The listing builds one solid part. Answer for the finished solid, in the listing's coordinates (mm). Coordinates: 2 decimals unless noted, no trailing zeros. Order: outer loops, then holes, each group sorted by start corner. A loop starts at its lowest first (then second) coordinate and runs counter-clockwise, first axis right, second up.
```python
from build123d import *

# Parameters (mm, degrees)
F0_R     = 3.175
F1_DEPTH = 6.35


with BuildPart() as f1:
    # F0 (on Top) → F1 (new body)
    with BuildSketch(Plane.XY):
        Polygon((0, 254), (0, 0), (53.975, 0), (53.975, 25.4), (73.025, 50.8), (73.025, 127), (485.775, 127), (485.775, 50.8), (504.825, 25.4), (504.825, 0), (558.8, 0), (558.8, 254), align=None)
        with Locations((12.7, 19.05)):
            Circle(F0_R, mode=Mode.SUBTRACT)
        with Locations((12.7, 63.5)):
            Circle(F0_R, mode=Mode.SUBTRACT)
        with Locations((11.1125, 107.95)):
            Circle(F0_R, mode=Mode.SUBTRACT)
        with Locations((549.275, 19.05)):
            Circle(F0_R, mode=Mode.SUBTRACT)
        with Locations((498.475, 76.2)):
            Circle(F0_R, mode=Mode.SUBTRACT)
        with Locations((549.275, 76.2)):
            Circle(F0_R, mode=Mode.SUBTRACT)
        with Locations((549.275, 107.95)):
            Circle(F0_R, mode=Mode.SUBTRACT)
        with Locations((523.875, 120.194091)):
            Circle(F0_R, mode=Mode.SUBTRACT)
        with Locations((9.525, 176.2125)):
            Circle(F0_R, mode=Mode.SUBTRACT)
        with Locations((60.325, 176.2125)):
            Circle(F0_R, mode=Mode.SUBTRACT)
        with Locations((92.075, 176.2125)):
            Circle(F0_R, mode=Mode.SUBTRACT)
        with Locations((142.875, 176.2125)):
            Circle(F0_R, mode=Mode.SUBTRACT)
        with Locations((34.925, 220.206591)):
            Circle(F0_R, mode=Mode.SUBTRACT)
        with Locations((117.475, 220.206591)):
            Circle(F0_R, mode=Mode.SUBTRACT)
        with Locations((381, 176.2125)):
            Circle(F0_R, mode=Mode.SUBTRACT)
        with Locations((431.8, 176.2125)):
            Circle(F0_R, mode=Mode.SUBTRACT)
        with Locations((461.9625, 176.2125)):
            Circle(F0_R, mode=Mode.SUBTRACT)
        with Locations((512.7625, 176.2125)):
            Circle(F0_R, mode=Mode.SUBTRACT)
        with Locations((406.4, 220.206591)):
            Circle(F0_R, mode=Mode.SUBTRACT)
        with Locations((461.9625, 204.7875)):
            Circle(F0_R, mode=Mode.SUBTRACT)
        with Locations((487.3625, 220.206591)):
            Circle(F0_R, mode=Mode.SUBTRACT)
        with Locations((512.7625, 204.7875)):
            Circle(F0_R, mode=Mode.SUBTRACT)
    extrude(amount=F1_DEPTH)


solid = f1.part
```
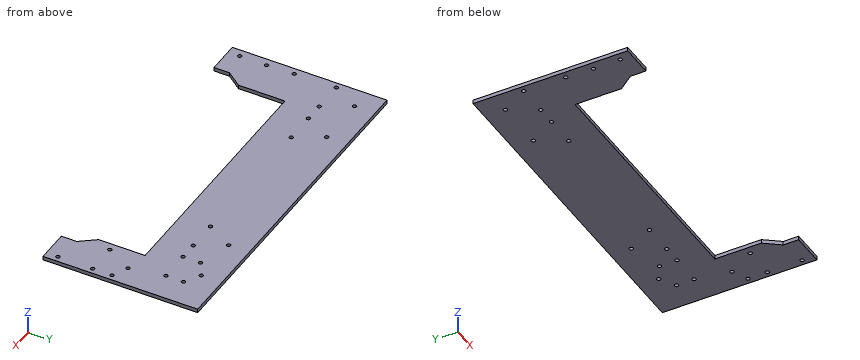
1) A cutting plane is placed at A-A, the plane y = 97.5. Write down the section's boundary in (x, z) (3 decimals).
2) A cutting plane is placed at B-B, the plane y = 32.5. Write down the section's boundary in (x, z), plus the area to 3 significant figures.
3) Straight lines are drawn through the part: probe 1 along X at (y, z) = (109.5, 0.75) (3 decimals); probe 2 along Y at (x, z) = (390, 2); probe 3 along Y at (x, z) = (381, 4.25). For each, find the intervals that lie inside material, in ascending order.
4) A cutting plane is placed at D-D, the plane x = 232.5. Write down the section's boundary in (y, z), plus the area to 3 significant figures.
5) A cutting plane is placed at C-C, the plane z = 2.75. Count the separate pieces of the cut face and the enclosed holes in it, plus the area to 3 significant figures.
6) This flat-tipped pin is pushed along its axis until it touches: P1, Ø2, axis at x = 241.5, z = 2.5, coming from the -Y side. Where does it stop, or does it pass through?
Working result:
1. outline: (0, 0) - (73.025, 0) - (73.025, 6.35) - (0, 6.35) - close; (485.775, 0) - (558.8, 0) - (558.8, 6.35) - (485.775, 6.35) - close
2. outline: (0, 0) - (59.3, 0) - (59.3, 6.35) - (0, 6.35) - close; (499.5, 0) - (558.8, 0) - (558.8, 6.35) - (499.5, 6.35) - close
2. area: 753 mm2
3. probe 1: x = 0 to 8.342, 13.883 to 73.025, 485.775 to 546.504, 552.046 to 558.8
3. probe 2: y = 127 to 254
3. probe 3: y = 127 to 173.04, 179.39 to 254
4. outline: (127, 0) - (254, 0) - (254, 6.35) - (127, 6.35) - close
4. area: 806 mm2
5. separate pieces: 1
5. enclosed holes: 22
5. area: 87,400 mm2
6. P1: stops at y = 127
